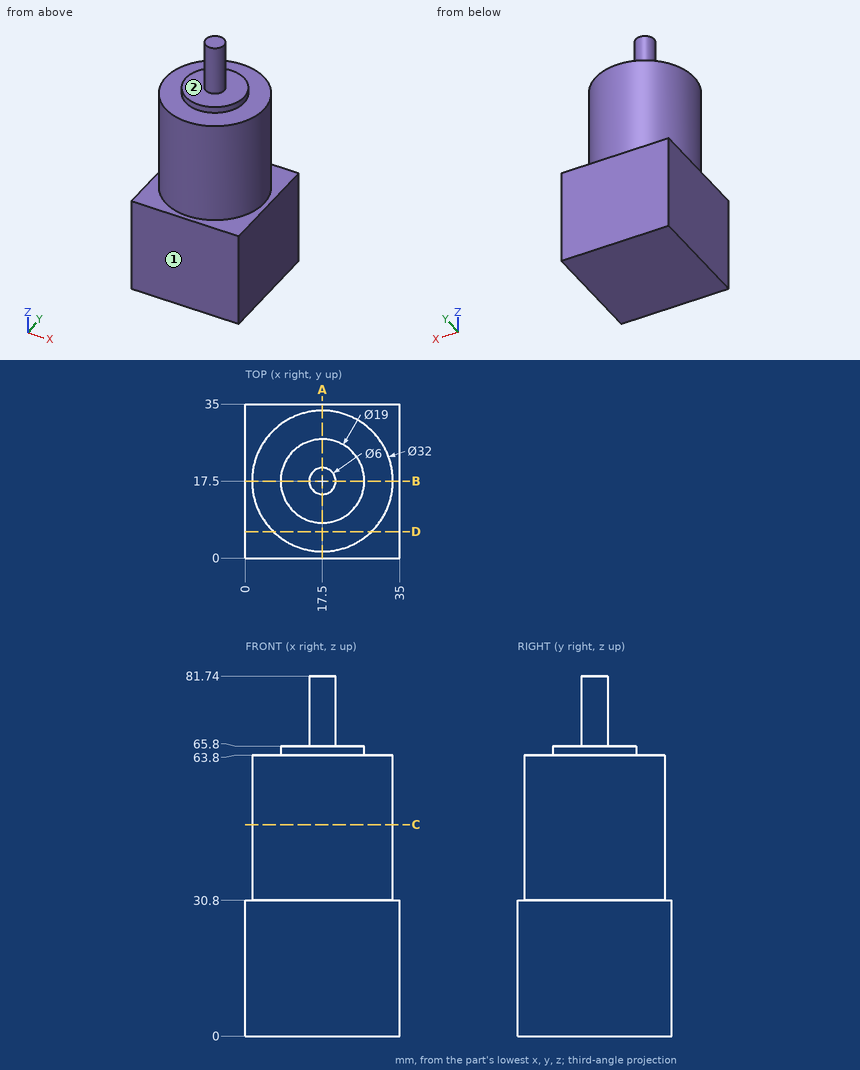
Geometry: see drawing. Coordinates: mm, zero at the bounding-box minimum. A direction names the side the tool comes from. Give positions to 0.01 mm unless a question says otherwise; leave off trailing zeros. Write each loop counter-clockwise with the first axis right and the second up, starting at its lowest first coordinate (ties: lowest second). Pieces come first, ordered by that corner, then holes. Notation, with made-up numbers: M 52,46.5 L 102,46.5 A21 cw 102,60.5 Z; hole C -24.5,34.5 d11. An arc over 180 degrees is marked long. Return JSON: item names as keys, results as strings. Group by question number.
1) Ray query, L1, parallel to Z at x = 13.5, y = 25; L2, parallel to Z at x = 31, y = 6; L3, parallel to Y at x = 18, z = 65.5. Return the intervals inside material, ascending.
2) Cut plane D-D, the plane y = 6. Output: boundary loops of the cut face in (x, z).
3) Cut plane A-A, the plane x = 17.5. Output: boundary loops of the cut face in (y, z).
4) Cut plane C-C, the plane z = 48. Output: boundary loops of the cut face in (x, y), then the cut area to 3 significant figures.
5) First-contact query: pin 1 Ø6 at (x, y) = (5, 10.5) entering from +Z; pin 2 Ø1 at (x, y) = (4, 29) entering from +Z; pin 3 Ø12 at (y, z) = (19.5, 72) entering from -X. Flat tips, straight axial feed; report the tip coordinate or a pass-through.
6) Set-up query: the marked faces 1 and 2. Return all of +Z, -Z, +X, -X, +Y, -Y with unobstructed straight access to the full face (end or side cutting, diameter ignored); none if empty.
Data:
{
 "1": {"L1": "z = 0 to 65.8", "L2": "z = 0 to 30.8", "L3": "y = 8.01 to 26.99"},
 "2": {"outline": "M 0,0 L 35,0 L 35,30.8 L 28.62,30.8 L 28.62,63.8 L 6.38,63.8 L 6.38,30.8 L 0,30.8 Z"},
 "3": {"outline": "M 0,0 L 35,0 L 35,30.8 L 33.5,30.8 L 33.5,63.8 L 27,63.8 L 27,65.8 L 20.5,65.8 L 20.5,81.74 L 14.5,81.74 L 14.5,65.8 L 8,65.8 L 8,63.8 L 1.5,63.8 L 1.5,30.8 L 0,30.8 Z"},
 "4": {"outline": "C 17.5,17.5 d32", "area": "804 mm²"},
 "5": {"pin 1": "stops at z = 63.8", "pin 2": "stops at z = 30.8", "pin 3": "stops at x = 14.5"},
 "6": {"face 1": "+Z, -Z, +X, -X, -Y", "face 2": "+Z"}
}
